Can you work these out from the drawing? Everything is in mm from the part's minimum corner. Round coordinates to 2 decimals unless told otherwise and drop trailing zeros. Write each loop counter-clockwise with the first axis right and the second up, starting at its lowest first coordinate (ties: lowest second). Pieces come first, ordered by that corner, then holes. Notation, with made-up numbers: (25.5, 10.5) -> (80.5, 10.5) arc R14 ccw to (80.5, 30.5) -> close; hole circle Ø9 at (72, 70.25). An arc over 180 degrees is marked (long way). Answer as CSV lines item,"result". Start each with the question number.
Q1. Imagine slicing it at B-B on x = 75. Please give me the cut outline in (y, z), and give its area (3 significant figures).
Q2. Will this pin go through, and if not, where does the flat tip stop? pin 1 Ø8 at (x, y) = (45, 10) entering from -Z.
Q3. If I drill on line 1 (X direction, y = 14, z = 4.25); line 2 (X direction, y = 13, z = 7); line 3 (Y direction, x = 15, z = 9.75), over which ranges is the centre line in solid material (lowest first)? Write a range as [from, to].
Q4. Imagine slicing it at C-C on y = 10. Please give me the cut outline in (x, z), and give its area (3 significant figures).
Q5. Imagine slicing it at D-D on x = 48. Please give me the cut outline in (y, z).
Q6. Imagine slicing it at A-A on z = 12. Please give me the cut outline in (x, y).
Q7. If we mould it in two halves opening along X, with no side actions, what happens to the marked faces 1, 2 and 3? For each: pulls with the +X half, pulls with the -X half, needs draft (parallel to the pull), parting line crosses it, or undercut.
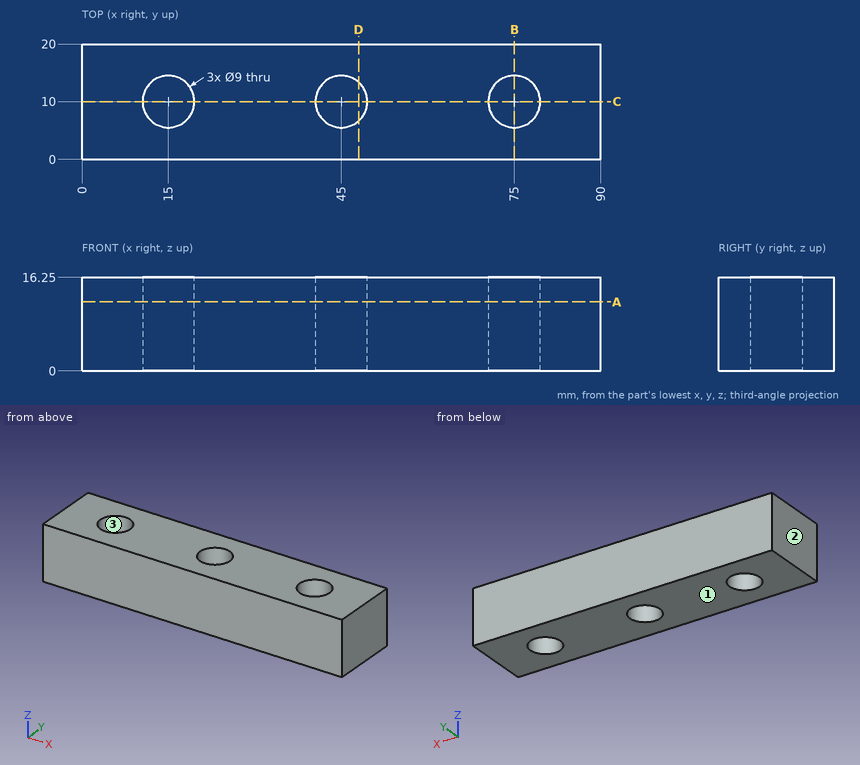
Checks:
1,outline,"(0, 0) -> (5.5, 0) -> (5.5, 16.25) -> (0, 16.25) -> close; (14.5, 0) -> (20, 0) -> (20, 16.25) -> (14.5, 16.25) -> close"
1,area,"179 mm^2"
2,pin 1,"through"
3,line 1,"[0, 12.94], [17.06, 42.94], [47.06, 72.94], [77.06, 90]"
3,line 2,"[0, 11.65], [18.35, 41.65], [48.35, 71.65], [78.35, 90]"
3,line 3,"[0, 5.5], [14.5, 20]"
4,outline,"(0, 0) -> (10.5, 0) -> (10.5, 16.25) -> (0, 16.25) -> close; (19.5, 0) -> (40.5, 0) -> (40.5, 16.25) -> (19.5, 16.25) -> close; (49.5, 0) -> (70.5, 0) -> (70.5, 16.25) -> (49.5, 16.25) -> close; (79.5, 0) -> (90, 0) -> (90, 16.25) -> (79.5, 16.25) -> close"
4,area,"1,020 mm^2"
5,outline,"(0, 0) -> (6.65, 0) -> (6.65, 16.25) -> (0, 16.25) -> close; (13.35, 0) -> (20, 0) -> (20, 16.25) -> (13.35, 16.25) -> close"
6,outline,"(0, 0) -> (90, 0) -> (90, 20) -> (0, 20) -> close; hole circle Ø9 at (15, 10); hole circle Ø9 at (45, 10); hole circle Ø9 at (75, 10)"
7,face 1,"needs draft"
7,face 2,"pulls with the -X half"
7,face 3,"undercut"
